Input: dimensioned drawing with shaded views. Units: mm. Origin: part minimum x, y, z. A direction names the side the tool comes from. Give positions to 0.01 mm unless a question says otherwise; leave off trailing zeros. Loops run counter-clockwise (first coordinate to the right, second up) from the corner with the lowest first, then second, coordinate; pieces in that order, holes last. Notation, with made-up numbers: (-14.5, 83.25) -> (21.5, 83.25) arc R12 cw to (21.5, 102.25) -> close; hole circle Ø11 at (36.5, 76.25). An arc over 180 degrees is marked (long way). Answer as a JSON object with one key per item and string values.
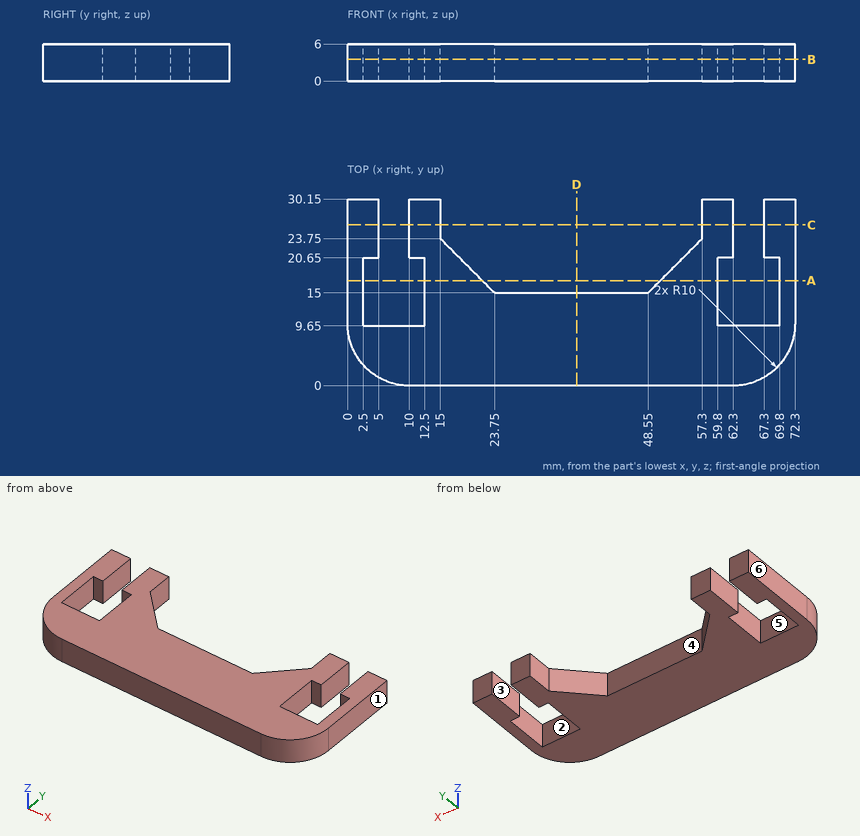
Q1. Section A-A, the plane y = 17. Return the cut outline in (x, z).
Evaluation:
{"outline": "(0, 0) -> (2.5, 0) -> (2.5, 6) -> (0, 6) -> close; (12.5, 0) -> (21.75, 0) -> (21.75, 6) -> (12.5, 6) -> close; (50.55, 0) -> (59.8, 0) -> (59.8, 6) -> (50.55, 6) -> close; (69.8, 0) -> (72.3, 0) -> (72.3, 6) -> (69.8, 6) -> close"}
Q2. Section D-D, the plane x = 37. Return the cut outline in (y, z), then the cut area to 3 significant figures.
Evaluation:
{"outline": "(0, 0) -> (15, 0) -> (15, 6) -> (0, 6) -> close", "area": "90.0 mm2"}
Q3. Ray query, line 1 along X through (y, z) = (14, 3); line 2 along X through (y, z) = (27, 1); line 3 along X through (y, z) = (17, 5.75). Return the intervals inside material, ascending.
Evaluation:
{"line 1": "x = 0 to 2.5, 12.5 to 59.8, 69.8 to 72.3", "line 2": "x = 0 to 5, 10 to 15, 57.3 to 62.3, 67.3 to 72.3", "line 3": "x = 0 to 2.5, 12.5 to 21.75, 50.55 to 59.8, 69.8 to 72.3"}
Q4. Section C-C, the plane y = 26. Return the cut outline in (x, z), then the cut area to 3 significant figures.
Evaluation:
{"outline": "(0, 0) -> (5, 0) -> (5, 6) -> (0, 6) -> close; (10, 0) -> (15, 0) -> (15, 6) -> (10, 6) -> close; (57.3, 0) -> (62.3, 0) -> (62.3, 6) -> (57.3, 6) -> close; (67.3, 0) -> (72.3, 0) -> (72.3, 6) -> (67.3, 6) -> close", "area": "120 mm2"}
Q5. Draft query along Y for the marked faces 4, 5 and 6. Return one class per face: +Y half, -Y half, draft (parallel to the pull), parting line (faces both ways), or undercut.
Evaluation:
{"face 4": "+Y half", "face 5": "undercut", "face 6": "draft"}
Q6. Access query for the marked faces 1, 2 and 3. Directions: +Z, -Z, +X, -X, +Y, -Y. A direction counts if a zero-diameter tool reaches every point of the face in a straight line with its end or side. Return the directions, or none.
Evaluation:
{"face 1": "+Z, -Z, +X, +Y, -Y", "face 2": "+Z, -Z", "face 3": "+Z, -Z, +Y"}
Q7. Section B-B, the plane z = 3.5. Return the cut outline in (x, y), then the cut area to 3 significant figures.
Evaluation:
{"outline": "(0, 10) arc R10 ccw to (10, 0) -> (62.3, 0) arc R10 ccw to (72.3, 10) -> (72.3, 30.15) -> (67.3, 30.15) -> (67.3, 20.65) -> (69.8, 20.65) -> (69.8, 9.65) -> (59.8, 9.65) -> (59.8, 20.65) -> (62.3, 20.65) -> (62.3, 30.15) -> (57.3, 30.15) -> (57.3, 23.75) -> (48.55, 15) -> (23.75, 15) -> (15, 23.75) -> (15, 30.15) -> (10, 30.15) -> (10, 20.65) -> (12.5, 20.65) -> (12.5, 9.65) -> (2.5, 9.65) -> (2.5, 20.65) -> (5, 20.65) -> (5, 30.15) -> (0, 30.15) -> close", "area": "1,260 mm2"}
Q8. Pin query (flat end, axial travel): pin 1 (1.8 mm diameter, centred on x = 8.5, z = 2, fed in from +Y); pin 2 (0.8 mm diameter, centred on x = 68, z = 2, fed in from -Y); pin 3 (1 mm diameter, centred on y = 4, z = 1, fed in from -X). Return the tip coordinate at first contact, or that it passes through.
Evaluation:
{"pin 1": "stops at y = 9.65", "pin 2": "stops at y = 1.52", "pin 3": "stops at x = 1.65"}
